Verification items for the finished model (mm, model axes). Face numbers are marked on the shaded views. A direction names the side the tool comes from. Round coordinates to 2 decimals unless told otherwise and drop trailing zeros. Write each loop counter-clockwise with the first axis right and the second up, starting at its lowest first coordinate (ties: lowest second). Pieces come first, ordered by that corner, then holes. Notation, with made-up numbers: (11, -24.5) -> (61, -24.5) arc R28 cw to (61, 12.5) -> close; hole circle Ø11 at (77, 69.5). An arc over 180 degrees is marked (long way). Answer as a JSON object with one key per item and string values. Group by question number.
(1) Sectioned sample at C-C on x = 2.25. Record the cut outline in (y, z), and give its area (3 significant figures).
(2) Sectioned sample at A-A on y = 0. Record the cut outline in (x, z).
(3) Scan lines: L1, parallel to X at y = 0, z = -13.25; L2, parallel to Z at x = -1.5, y = 8; L3, parallel to Y at x = -6, z = 8. Record each from-to range of solid material in increasing order. Write a range as from..to.
(4) Gauge pin test, flat ends, axial feed: pin 1 Ø3 at (x, z) = (0.5, 7) entering from -Y; pin 2 Ø4 at (x, y) = (0, -5) entering from +Z; pin 3 Ø4 at (x, y) = (-1.5, 5) entering from +Z. Record the tip position at first contact, or that the pin passes through.
(5) Set-up check for the marked faces 1 and 2: record each of +Z, -Z, +X, -X, +Y, -Y from which the full face is reachable in a straight line by a thin tool's end or side.
(6) Draft check along Y on the marked faces 3, 4 and 5. Enter one of: released by +Y, released by -Y, zero draft, split by the parting line, or undercut.
(7) Sectioned sample at D-D on x = -8.5. Record the cut outline in (y, z).
Autodesk Inventor part; units mm, degrees
ref_plane "YZ Plane" through (0, 0, 0) normal (1, 0, 0) x (0, 1, 0)
ref_plane "XZ Plane" through (0, 0, 0) normal (0, 1, 0) x (-1, 0, 0)
ref_plane "XY Plane" through (0, 0, 0) normal (0, 0, 1) x (1, 0, 0)
sketch "Sketch1" plane through (0, 0, 0) normal (0, 0, 1) x (1, 0, 0)
  line L0 (5, 0) -> (-5, 0)
  line L1 (-4.9655, 15) -> (-4.9655, 5)
  line L2 (-4.9655, 5) -> (5.0345, 5)
  line L3 (5.0345, 5) -> (5.0345, 15)
  line L4 (5.0345, 15) -> (4.0026, 15)
  line L5 (4.0026, 15) -> (2.8501, 13.0635)
  arc A0 (-2.8501, 13.0635) -> (2.8501, 13.0635) centre (0, 14) ccw
  line L6 (-2.8501, 13.0635) -> (-3.9336, 15)
  line L7 (-3.9336, 15) -> (-4.9655, 15)
  line L8 (-4.9655, 15) -> (-9.9655, 15)
  line L9 (-9.9655, 15) -> (-9.9655, 5)
  line L10 (-9.9655, 5) -> (-4.9655, 5)
  line L11 (0, 11) -> (0, 14)
  line L12 (0, 14) -> (0, 15)
  line L13 (0, 15) -> (4.0026, 15)
  point P0 (0, 0)
  dimension "d12" = 10
  dimension "d13" = 10
  dimension "d14" = 5
  dimension "d15" = 143.621
  dimension "d16" = 3
  dimension "d17" = 1.0319
  dimension "d18" = 1.0319
  dimension "d20" = 1
  dimension "d22" = 1.9365
  dimension "d23" = 4.0026
revolve "Revolution1" add sketch "Sketch1" angle 360 about axis through (5, 0, 0) along (-1, 0, 0) contours L7 L6 A0 L5 L4 L3 L2 L1 | L1 L10 L9 L8
sketch "Sketch2" plane through (5.0345, 0, 0) normal (1, 0, 0) x (0, 0, -1)
  circle A0 centre (0, 0) radius 5
  circle A1 centre (0, 0) radius 8
  line L0 (-8, 0) -> (8, 0)
  dimension "d1" = 16
hole "Hole1" at (5.0345, 0, 8) direction (-1, 0, 0) diameter 2 end through all
pattern_circular "Circular Pattern1" count 4 over 360 about axis through (-7.4655, 0, 0) along (1, 0, 0) of "Hole1"
properties part number "motor_trinse"
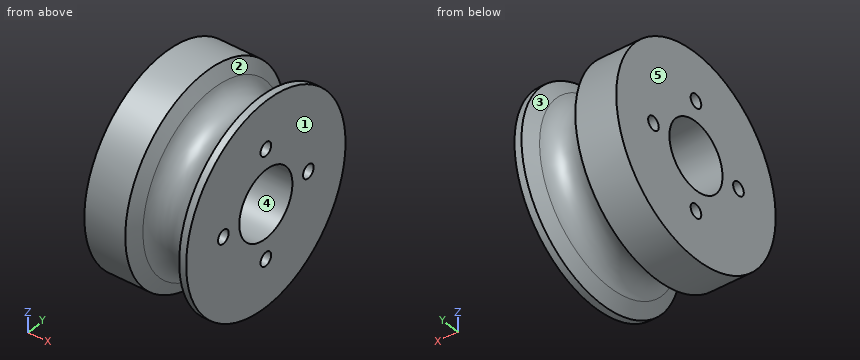
Computed values:
{
 "1": {"outline": "circle Ø24.03 at (0, 0); hole circle Ø2 at (-8, 0); hole circle Ø10 at (0, 0); hole circle Ø2 at (0, -8); hole circle Ø2 at (0, 8); hole circle Ø2 at (8, 0)", "area": "362 mm2"},
 "2": {"outline": "(-9.97, -15) -> (-3.93, -15) -> (-2.85, -13.06) arc R3 cw to (2.85, -13.06) -> (4, -15) -> (5.03, -15) -> (5.03, -9) -> (-9.97, -9) -> close; (-9.97, -7) -> (5.03, -7) -> (5.03, -5) -> (-9.97, -5) -> close; (-9.97, 5) -> (5.03, 5) -> (5.03, 7) -> (-9.97, 7) -> close; (-9.97, 9) -> (5.03, 9) -> (5.03, 15) -> (4, 15) -> (2.85, 13.06) arc R3 cw to (-2.85, 13.06) -> (-3.93, 15) -> (-9.97, 15) -> close"},
 "3": {"L1": "-9.97..-2.95, 2.96..5.03", "L2": "-8.12..-1, 1..8.12", "L3": "-12.69..-1, 1..12.69"},
 "4": {"pin 1": "y = -9.78", "pin 2": "z = 10.84", "pin 3": "z = 13.39"},
 "5": {"face 1": "+Z, -Z, +X, +Y, -Y", "face 2": "none"},
 "6": {"face 3": "split by the parting line", "face 4": "undercut", "face 5": "zero draft"},
 "7": {"outline": "circle Ø30 at (0, 0); hole circle Ø2 at (-8, 0); hole circle Ø10 at (0, 0); hole circle Ø2 at (0, -8); hole circle Ø2 at (0, 8); hole circle Ø2 at (8, 0)"}
}
